The drawing under review shows one solid part. Ordinate dimensions are in mm from its lowest x, y, z. A direction names the side the tool comes from. Coordinates: 2 decimals unless noted, no trailing zeros. Loops run counter-clockwise (first coordinate to the right, second up) from the corner with the lowest first, then second, coordinate; pieces in that order, holes last. Notation, with made-up numbers: M 50,62.25 L 96,62.25 A25 ccw 96,92.25 Z; hole C 88.25,-36 d7. An arc over 180 degrees is marked long. Put each result on its own line as item: value.
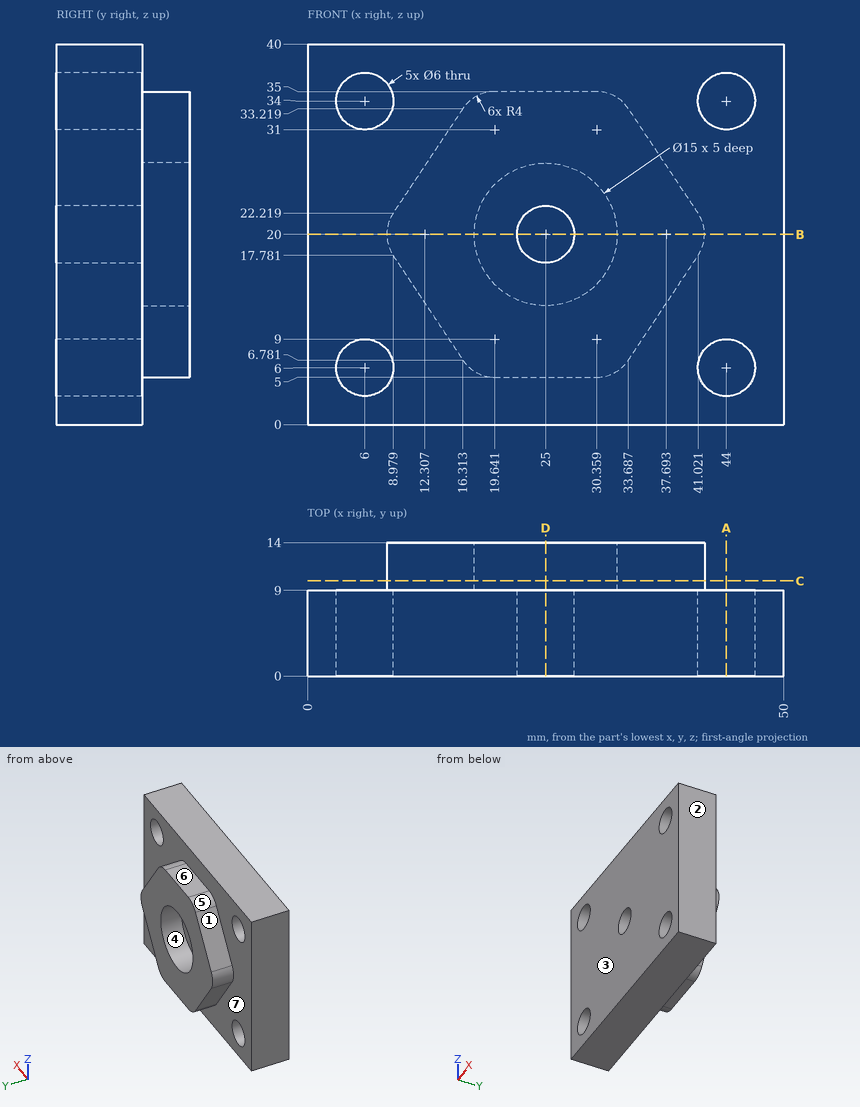
(1) Add section C-C (y = 10). Write out the cut boundary in (x, z), plus the area to 3 significant figures.
Determined:
outline: M 8.98,17.78 L 16.31,6.78 A4 ccw 19.64,5 L 30.36,5 A4 ccw 33.69,6.78 L 41.02,17.78 A4 ccw 41.02,22.22 L 33.69,33.22 A4 ccw 30.36,35 L 19.64,35 A4 ccw 16.31,33.22 L 8.98,22.22 A4 ccw Z; hole C 25,20 d15
area: 568 mm^2
(2) Draft analysis for pull direction X (two halves, no side actions). For the marked faces 1, 2, 3 and 4, state which applies: +X half, -X half, draft (parallel to the pull), parting line (faces both ways), or undercut.
Determined:
face 1: -X half
face 2: +X half
face 3: draft
face 4: undercut
(3) Tool access review of the marked faces 5, 6 and 7: name each direction out of +Z, -Z, +X, -X, +Y, -Y from which nothing blocks a thin tool from reaching the whole face with its end or side.
Determined:
face 5: +Z, -X, +Y
face 6: +Z, +X, -X, +Y
face 7: +Y
(4) Add section D-D (x = 25). Write out the cut boundary in (y, z), plus the area to 3 significant figures.
Determined:
outline: M 0,0 L 9,0 L 9,5 L 14,5 L 14,12.5 L 9,12.5 L 9,17 L 0,17 Z; M 0,23 L 9,23 L 9,27.5 L 14,27.5 L 14,35 L 9,35 L 9,40 L 0,40 Z
area: 381 mm^2
(5) For pin 1 (5 mm diameter, centred on x = 44, z = 6, fed in from +Y); pin 2 (2 mm diameter, centred on y = 12, z = 9, fed in from -X); pin 3 (2.5 mm diameter, centred on x = 22.5, y = 11.5, fed in from +Z); pin 4 (9.5 mm diameter, centred on x = 44, z = 34, fed in from +Y), all flat-tipped, find the tip position at first contact; note any pin that passes through.
Determined:
pin 1: passes through
pin 2: stops at x = 14.17
pin 3: stops at z = 35
pin 4: stops at y = 9
(6) Add section A-A (x = 44). Write out the cut boundary in (y, z).
Determined:
outline: M 0,0 L 9,0 L 9,3 L 0,3 Z; M 0,9 L 9,9 L 9,31 L 0,31 Z; M 0,37 L 9,37 L 9,40 L 0,40 Z
(7) Add section B-B (z = 20). Write out the cut boundary in (x, y).
Determined:
outline: M 0,0 L 22,0 L 22,9 L 17.5,9 L 17.5,14 L 8.31,14 L 8.31,9 L 0,9 Z; M 28,0 L 50,0 L 50,9 L 41.69,9 L 41.69,14 L 32.5,14 L 32.5,9 L 28,9 Z
(8) Wall thickness on line 1 along X through (y, z) = (3.75, 34); line 2 along X through (y, z) = (1.5, 35); line 3 along X through (y, z) = (11.15, 20): over which ranges is each line inside the solid? List them lowest first. Write a range as [from, to].
Determined:
line 1: x = [0, 3], [9, 41], [47, 50]
line 2: x = [0, 3.17], [8.83, 41.17], [46.83, 50]
line 3: x = [8.31, 17.5], [32.5, 41.69]
